Check sheet for the modelled part. Datum: model origin and axes. Units: mm. Give positions to 0.01 mm unless a question says otherwise; leave off trailing zeros. Write each loop counter-clockwise with the first axis right and the second up, starting at its lowest first coordinate (ties: lowest second). Pieces come first, ordered by that corner, then holes. Notation, with made-up numbers: M 63.5,66 L 111.5,66 A27 ccw 111.5,84 Z; hole C 37,24.5 d6. An arc over 180 degrees is marked long. Use CSV: the item, a comma, the result in double quotes. Start each with the question number.
1. Depth check by flat-ended pin: P1, Ø19.5, axis at x = 32.23, z = -10.21, coming from the -Y side. Enter the tip coordinate at first touch or a pass-through.
2. Cross-section at C-C, the plane z = -1.5. Enter the section's corners in (x, y).
3. Mould release check, pull along X, two halves, no side actions. Record for faces 1 (the face through (37, -0.75, -17)), 2 (the face through (-0.432, -0.74, 14.248)), 3 (the face through (39.155, -0.37, -13.077)): +X half, -X half, draft (parallel to the pull), parting line (faces both ways), or undercut.
4. Scan lines: line 1 (X direction, y = -1, z = -5.5); line 2 (X direction, y = -0.4, z = -15.5); line 3 (X direction, y = -0.2, z = -15). Record each from-to range of solid material in increasing order.
5. Cross-section at A-A, the plane x = 35.5. Enter the section's corners in (y, z).
6. Cross-section at D-D, the plane y = -0.35. Enter the section's corners in (x, z), and give its area (3 significant figures).
7. Cross-section at B-B, the plane z = -9. Enter the section's corners in (x, y).
from build123d import *

# Parameters (mm, degrees)
F1_DEPTH = 1.5
F0_W     = 21.057298
F0_H     = 23.743179
F0_R     = 7.495866
F2_DEPTH = 0.75


with BuildPart() as f1:
    # F0 (on Front) → F1 (new body)
    with BuildSketch(Plane.XZ):
        Polygon((-23.635745, 28.90007), (-45.122784, 28.90007), (-45.122784, -23.743179), (22.131654, -23.743179), (22.131654, 0), align=None)
    extrude(amount=F1_DEPTH)

    # F0 (on Front) → F2 (join)
    with BuildSketch(Plane.XZ):
        Polygon((-23.635745, 28.90007), (-45.122784, 28.90007), (-45.122784, -23.743179), (22.131654, -23.743179), (22.131654, 0), align=None)
        with Locations((32.660303, -11.871589)):
            Rectangle(F0_W, F0_H)
        with Locations((32.23056, -10.206345)):
            Circle(F0_R, mode=Mode.SUBTRACT)
    extrude(amount=F2_DEPTH)


solid = f1.part
Worked answers:
1,P1,"stops at y = -0.75"
2,outline,"M -45.12,-1.5 L 22.13,-1.5 L 22.13,-0.75 L 43.19,-0.75 L 43.19,0 L -45.12,0 Z"
3,face 1,"draft"
3,face 2,"+X half"
3,face 3,"undercut"
4,line 1,"x = -45.12 to 22.13"
4,line 2,"x = -45.12 to 26.92, 37.54 to 43.19"
4,line 3,"x = -45.12 to 26.47, 37.99 to 43.19"
5,outline,"M -0.75,-23.74 L 0,-23.74 L 0,-16.95 L -0.75,-16.95 Z; M -0.75,-3.46 L 0,-3.46 L 0,0 L -0.75,0 Z"
6,outline,"M -45.12,-23.74 L 43.19,-23.74 L 43.19,0 L 22.13,0 L -23.64,28.9 L -45.12,28.9 Z; hole C 32.23,-10.21 d14.99"
6,area,"3,200 mm^2"
7,outline,"M -45.12,-1.5 L 22.13,-1.5 L 22.13,-0.75 L 24.83,-0.75 L 24.83,0 L -45.12,0 Z; M 39.63,-0.75 L 43.19,-0.75 L 43.19,0 L 39.63,0 Z"
